from build123d import *

# Parameters (mm, degrees)
SKETCH1_W                = 105
SKETCH1_H                = 90
BOSS_EXTRUDE1_DEPTH      = 2
M3_CLEARANCE_HOLE1_D     = 3
M3_CLEARANCE_HOLE1_DEPTH = 2
M3_CLEARANCE_HOLE1_TIP   = 0.901290929
SKETCH4_W                = 4
SKETCH4_H                = 3
CUT_EXTRUDE1_DEPTH       = 139.307628134
FILLET1_R                = 1
FILLET2_R                = 1
FILLET3_R                = 1
FILLET4_R                = 1
LPATTERN1_COUNT          = 2
LPATTERN1_PITCH          = 75
LPATTERN1_COUNT_DIR2     = 3
LPATTERN1_PITCH_DIR2     = 38
FILLET1_OF_LPATTERN1_R   = 1
FILLET2_OF_LPATTERN1_R   = 1
FILLET3_OF_LPATTERN1_R   = 1
FILLET4_OF_LPATTERN1_R   = 1
CUT_EXTRUDE2_DEPTH       = 139.307628134


with BuildPart() as part:
    # Sketch1 → Boss-Extrude1 (new body)
    with BuildSketch(Plane(origin=(0, 0, 0), x_dir=(1, 0, 0), z_dir=(0, 1, 0))):
        with Locations((52.5, 45)):
            Rectangle(SKETCH1_W, SKETCH1_H)
    extrude(amount=BOSS_EXTRUDE1_DEPTH)

    # M3 Clearance Hole1
    with Locations(Plane(origin=(0, 2, 0), x_dir=(1, 0, 0), z_dir=(0, 1, 0))):
        with Locations((5.46, 11.98), (5.46, 78.02), (99.54, 78.02), (99.54, 11.98)):
            Hole(M3_CLEARANCE_HOLE1_D / 2, depth=M3_CLEARANCE_HOLE1_DEPTH)
            with Locations((0, 0, -(M3_CLEARANCE_HOLE1_DEPTH + M3_CLEARANCE_HOLE1_TIP / 2))):  # 118° drill point
                Cone(0, M3_CLEARANCE_HOLE1_D / 2, M3_CLEARANCE_HOLE1_TIP, mode=Mode.SUBTRACT)

    # Sketch4 → Cut-Extrude1 (cut, through all)
    with BuildSketch(Plane(origin=(0, 2, 0), x_dir=(1, 0, 0), z_dir=(0, 1, 0))):
        with Locations((14.5, 82.5)):
            Rectangle(SKETCH4_W, SKETCH4_H)
    cut_extrude1 = extrude(amount=-CUT_EXTRUDE1_DEPTH, mode=Mode.SUBTRACT)

    # Fillet1
    fillet1_edges = [part.edges().sort_by_distance(p)[0] for p in [
        (12.5, 1, -84),
    ]]
    fillet(fillet1_edges, radius=FILLET1_R)

    # Fillet2
    fillet2_edges = [part.edges().sort_by_distance(p)[0] for p in [
        (12.5, 1, -81),
    ]]
    fillet(fillet2_edges, radius=FILLET2_R)

    # Fillet3
    fillet3_edges = [part.edges().sort_by_distance(p)[0] for p in [
        (16.5, 1, -84),
    ]]
    fillet(fillet3_edges, radius=FILLET3_R)

    # Fillet4
    fillet4_edges = [part.edges().sort_by_distance(p)[0] for p in [
        (16.5, 1, -81),
    ]]
    fillet(fillet4_edges, radius=FILLET4_R)

    # LPattern1: Cut-Extrude1 2 × 3
    with Locations(*[(j * LPATTERN1_PITCH_DIR2, 0, i * LPATTERN1_PITCH) for i in range(LPATTERN1_COUNT) for j in range(LPATTERN1_COUNT_DIR2) if (i, j) != (0, 0)]):
        add(cut_extrude1, mode=Mode.SUBTRACT)

    # Fillet1 of LPattern1
    fillet1_of_lpattern1_edges = [part.edges().sort_by_distance(p)[0] for p in [
        (50.5, 1, -84),
        (88.5, 1, -84),
        (12.5, 1, -9),
        (50.5, 1, -9),
        (88.5, 1, -9),
    ]]
    fillet(fillet1_of_lpattern1_edges, radius=FILLET1_OF_LPATTERN1_R)

    # Fillet2 of LPattern1
    fillet2_of_lpattern1_edges = [part.edges().sort_by_distance(p)[0] for p in [
        (50.5, 1, -81),
        (88.5, 1, -81),
        (12.5, 1, -6),
        (50.5, 1, -6),
        (88.5, 1, -6),
    ]]
    fillet(fillet2_of_lpattern1_edges, radius=FILLET2_OF_LPATTERN1_R)

    # Fillet3 of LPattern1
    fillet3_of_lpattern1_edges = [part.edges().sort_by_distance(p)[0] for p in [
        (54.5, 1, -84),
        (92.5, 1, -84),
        (16.5, 1, -9),
        (54.5, 1, -9),
        (92.5, 1, -9),
    ]]
    fillet(fillet3_of_lpattern1_edges, radius=FILLET3_OF_LPATTERN1_R)

    # Fillet4 of LPattern1
    fillet4_of_lpattern1_edges = [part.edges().sort_by_distance(p)[0] for p in [
        (54.5, 1, -81),
        (92.5, 1, -81),
        (16.5, 1, -6),
        (54.5, 1, -6),
        (92.5, 1, -6),
    ]]
    fillet(fillet4_of_lpattern1_edges, radius=FILLET4_OF_LPATTERN1_R)

    # Sketch6 → Cut-Extrude2 (cut, through all)
    with BuildSketch(Plane.XZ):
        with BuildLine():
            Line((31.726499367, -27.824570361), (35.324813273, -24.217791062))
            ThreePointArc((35.324813273, -24.217791062), (38.153238445, -24.214467895), (38.156561613, -27.042893068))
            Line((38.156561613, -27.042893068), (34.558247707, -30.649672366))
            ThreePointArc((34.558247707, -30.649672366), (31.729822534, -30.652995533), (31.726499367, -27.824570361))
        make_face()
        with BuildLine():
            Line((45.144836896, -34.196957958), (41.658406286, -37.691590744))
            ThreePointArc((41.658406286, -37.691590744), (38.829981114, -37.694913911), (38.826657946, -34.866488738))
            Line((38.826657946, -34.866488738), (42.313088556, -31.371855953))
            ThreePointArc((42.313088556, -31.371855953), (45.141513729, -31.368532786), (45.144836896, -34.196957958))
        make_face()
        with BuildLine():
            Line((69.676107758, -65.774178752), (73.282887056, -62.175864846))
            ThreePointArc((73.282887056, -62.175864846), (73.286210223, -59.347439673), (70.457785051, -59.344116506))
            Line((70.457785051, -59.344116506), (66.851005753, -62.942430412))
            ThreePointArc((66.851005753, -62.942430412), (66.847682586, -65.770855585), (69.676107758, -65.774178752))
        make_face()
        with BuildLine():
            Line((63.30372016, -52.355841223), (59.809087375, -55.842271833))
            ThreePointArc((59.809087375, -55.842271833), (59.805764208, -58.670697005), (62.63418938, -58.674020172))
            Line((62.63418938, -58.674020172), (66.128822166, -55.187589562))
            ThreePointArc((66.128822166, -55.187589562), (66.132145333, -52.35916439), (63.30372016, -52.355841223))
        make_face()
        with BuildLine():
            Line((99.169047558, -33.68696962), (91.390872965, -41.465144213))
            ThreePointArc((91.390872965, -41.465144213), (88.562445841, -41.465144213), (88.562445841, -38.636717088))
            Line((88.562445841, -38.636717088), (96.340620434, -30.858542495))
            ThreePointArc((96.340620434, -30.858542495), (99.169047558, -30.858542495), (99.169047558, -33.68696962))
        make_face()
        with BuildLine():
            Line((16.492855818, -51.419940807), (8.714681224, -59.1981154))
            ThreePointArc((8.714681224, -59.1981154), (5.8862541, -59.1981154), (5.8862541, -56.369688276))
            Line((5.8862541, -56.369688276), (13.664428693, -48.591513683))
            ThreePointArc((13.664428693, -48.591513683), (16.492855818, -48.591513683), (16.492855818, -51.419940807))
        make_face()
        with BuildLine():
            Line((16.492855818, -65.562076431), (18.455777203, -63.599155046))
            ThreePointArc((18.455777203, -63.599155046), (21.284204328, -63.599155046), (21.284204328, -66.42758217))
            Line((21.284204328, -66.42758217), (19.321282942, -68.390503556))
            ThreePointArc((19.321282942, -68.390503556), (16.492855818, -68.390503556), (16.492855818, -65.562076431))
        make_face()
        with BuildLine():
            Line((88.562445841, -24.494581464), (85.734018716, -27.323008589))
            ThreePointArc((85.734018716, -27.323008589), (82.905591591, -27.323008589), (82.905591591, -24.494581464))
            Line((82.905591591, -24.494581464), (85.734018716, -21.666154339))
            ThreePointArc((85.734018716, -21.666154339), (88.562445841, -21.666154339), (88.562445841, -24.494581464))
        make_face()
        with BuildLine():
            Line((34.618363651, -60.312489091), (37.188189027, -62.882314467))
            ThreePointArc((37.188189027, -62.882314467), (37.188189027, -65.710741592), (34.359761903, -65.710741592))
            Line((34.359761903, -65.710741592), (31.789936526, -63.140916216))
            ThreePointArc((31.789936526, -63.140916216), (31.789936526, -60.312489091), (34.618363651, -60.312489091))
        make_face()
        with BuildLine():
            Line((67.811810973, -27.11904177), (70.381636349, -29.688867146))
            ThreePointArc((70.381636349, -29.688867146), (73.210063474, -29.688867146), (73.210063474, -26.860440021))
            Line((73.210063474, -26.860440021), (70.640238097, -24.290614645))
            ThreePointArc((70.640238097, -24.290614645), (67.811810973, -24.290614645), (67.811810973, -27.11904177))
        make_face()
        with BuildLine():
            Line((40.278245356, -54.658662907), (42.845042972, -57.225460523))
            ThreePointArc((42.845042972, -57.225460523), (42.845042972, -60.053887648), (40.016615847, -60.053887648))
            Line((40.016615847, -60.053887648), (37.449818231, -57.487090032))
            ThreePointArc((37.449818231, -57.487090032), (37.449818231, -54.658662907), (40.278245356, -54.658662907))
        make_face()
        with BuildLine():
            Line((62.157984789, -32.778923475), (64.724782404, -35.345721091))
            ThreePointArc((64.724782404, -35.345721091), (67.553209529, -35.345721091), (67.553209529, -32.517293966))
            Line((67.553209529, -32.517293966), (64.986411913, -29.95049635))
            ThreePointArc((64.986411913, -29.95049635), (62.157984789, -29.95049635), (62.157984789, -32.778923475))
        make_face()
    extrude(amount=-CUT_EXTRUDE2_DEPTH, mode=Mode.SUBTRACT)


solid = part.part
The listing builds one solid part. Answer for the finished solid, in the listing's coordinates (mm). Give positions to 0.01 mm unless a question says otherwise; leave off trailing zeros. Order: outer loops, then holes, each group sorted by start corner. A loop starts at its lowest first (then second) coordinate and runs counter-clockwise, first axis right, second up. Notation, with made-up numbers: (-10.75, 49.25) -> (36.25, 49.25) arc R7 ccw to (36.25, 55.25) -> close; hole circle Ø9 at (52, -17). An arc over 180 degrees is marked (long way). Put each result on its own line as item: value.
Item 1: A cutting plane is placed at A-A on z = -11.98. Give the vertices of the cut face in (x, y), plus the area to 3 significant figures.
Established:
outline: (0, 0) -> (3.96, 0) -> (3.96, 2) -> (0, 2) -> close; (6.96, 0) -> (98.04, 0) -> (98.04, 2) -> (6.96, 2) -> close; (101.04, 0) -> (105, 0) -> (105, 2) -> (101.04, 2) -> close
area: 198 mm^2
Item 2: A cutting plane is placed at C-C on y = 0.65. Count the separate pieces of the cut face and the enclosed holes in it, plus the area to 3 significant figures.
Established:
separate pieces: 1
enclosed holes: 22
area: 8,950 mm^2
Item 3: A cutting plane is placed at B-B on x = 11. Give the vertices of the cut face in (y, z).
Established:
outline: (0, -90) -> (2, -90) -> (2, -56.91) -> (0, -56.91) -> close; (0, -51.26) -> (2, -51.26) -> (2, 0) -> (0, 0) -> close
Item 4: Straight lines are drawn through the part: line 1 (X direction, y = 0.55, z = -11.98); line 2 (Z direction, x = 99.54, y = 0.55); line 3 (Z direction, x = 99.5, y = 0.8). For each, find the intervals that lie inside material, in ascending order.
Established:
line 1: x = 0 to 3.96, 6.96 to 98.04, 101.04 to 105
line 2: z = -90 to -79.52, -76.52 to -33.17, -31.37 to -13.48, -10.48 to 0
line 3: z = -90 to -79.52, -76.52 to -33.25, -31.3 to -13.48, -10.48 to 0
Item 5: For a pull along Z with two mould halves and no side action, classify faces 1 (the face through (52, 0, -46)), 2 (the face through (66.16, 0.99, -52.39)) as released by +Z, released by -Z, zero draft, split by the parting line, or undercut.
Established:
face 1: zero draft
face 2: undercut
Item 6: Given P1, Ø1.1, axis at y = 1, z = -82.5, coming from the -X side, flat-ended and moving along its own axis, determine where the tip first touches the part or whether it passes through.
Established:
P1: stops at x = 0
